```python
from build123d import *

# Parameters (mm, degrees)
SKETCH2_R            = 39.5
BOSS_EXTRUDE1_DEPTH  = 1
SKETCH4_R            = 41.25
BOSS_EXTRUDE2_DEPTH  = 0.7
SKETCH5_R            = 42
BOSS_EXTRUDE3_DEPTH  = 7
SKETCH6_R            = 35
BOSS_EXTRUDE4_DEPTH  = 3
SKETCH7_R            = 2.959266208
BOSS_EXTRUDE5_DEPTH  = 2.7
SKETCH8_R            = 2.259266208
CUT_EXTRUDE1_DEPTH   = 0.5
CIRPATTERN1_COUNT    = 12
SKETCH9_W            = 24
SKETCH9_H            = 40
BOSS_EXTRUDE6_DEPTH  = 42
BOSS_EXTRUDE7_DEPTH  = 24
SKETCH13_R           = 10
BOSS_EXTRUDE10_DEPTH = 10
SKETCH14_R           = 10
BOSS_EXTRUDE11_DEPTH = 10


with BuildPart() as part:
    # Sketch1 → Revolve1 (revolve)
    with BuildSketch(Plane.XY, mode=Mode.PRIVATE) as revolve1_sk:
        with BuildLine():
            Line((0, 0), (-35, 0))
            ThreePointArc((-35, 0), (-39.657515479, -9.46062113), (-40, -20))
            Line((-40, -20), (0, -20))
            Line((0, -20), (0, 0))
        make_face()
    revolve(revolve1_sk.sketch.rotate(Axis((0, 0, 0), (0, -1, 0)), 270), axis=Axis((0, 0, 0), (0, -1, 0)))

    # Sketch2 → Boss-Extrude1 (add)
    with BuildSketch(Plane.XZ.offset(20)):
        with Locations(Location((0, 0, 0), (0, 0, 270))):
            Circle(SKETCH2_R)
    extrude(amount=BOSS_EXTRUDE1_DEPTH)

    # Sketch3 → Revolve2 (revolve)
    with BuildSketch(Plane.XY, mode=Mode.PRIVATE) as revolve2_sk:
        with BuildLine():
            Line((0, -21), (-40, -21))
            ThreePointArc((-40, -21), (-42.384109041, -30.861589096), (-42, -41))
            Line((-42, -41), (0, -41))
            Line((0, -41), (0, -21))
        make_face()
    revolve(revolve2_sk.sketch.rotate(Axis((0, -21, 0), (0, -1, 0)), 270), axis=Axis((0, -21, 0), (0, -1, 0)))

    # Sketch4 → Boss-Extrude2 (add)
    with BuildSketch(Plane.XZ.offset(41)):
        Circle(SKETCH4_R)
    extrude(amount=BOSS_EXTRUDE2_DEPTH)

    # Sketch5 → Boss-Extrude3 (add)
    with BuildSketch(Plane.XZ.offset(41.7)):
        Circle(SKETCH5_R)
    extrude(amount=BOSS_EXTRUDE3_DEPTH)

    # Sketch6 → Boss-Extrude4 (add)
    with BuildSketch(Plane.XZ.offset(48.7)):
        Circle(SKETCH6_R)
    extrude(amount=BOSS_EXTRUDE4_DEPTH)

    # Sketch7 → Boss-Extrude5 (add)
    with BuildSketch(Plane.XZ.offset(48.7)):
        with Locations(Location((38.5, 0, 0), (0, 0, 180))):
            Circle(SKETCH7_R)
    boss_extrude5 = extrude(amount=BOSS_EXTRUDE5_DEPTH)

    # Sketch8 → Cut-Extrude1 (cut)
    with BuildSketch(Plane.XZ.offset(51.4)):
        with Locations((38.5, 0)):
            Circle(SKETCH8_R)
    cut_extrude1 = extrude(amount=-CUT_EXTRUDE1_DEPTH, mode=Mode.SUBTRACT)

    # CirPattern1: Boss-Extrude5, Cut-Extrude1 ×12 about axis
    cirpattern1_axis = Axis((0, 0, 0), (0, 1, 0))
    add([boss_extrude5.rotate(cirpattern1_axis, i * 360 / CIRPATTERN1_COUNT) for i in range(1, CIRPATTERN1_COUNT)])
    add([cut_extrude1.rotate(cirpattern1_axis, i * 360 / CIRPATTERN1_COUNT) for i in range(1, CIRPATTERN1_COUNT)], mode=Mode.SUBTRACT)

    # Sketch9 → Boss-Extrude6 (add)
    with BuildSketch(Plane(origin=(0, 0, 0), x_dir=(1, 0, 0), z_dir=(0, 1, 0))):
        Rectangle(SKETCH9_W, SKETCH9_H)
    extrude(amount=BOSS_EXTRUDE6_DEPTH)

    # Sketch10 → Boss-Extrude7 (add)
    with BuildSketch(Plane(origin=(12, 0, 0), x_dir=(0, 0, -1), z_dir=(1, 0, 0))):
        with BuildLine():
            Line((-20, 42), (20, 42))
            ThreePointArc((20, 42), (0, 62), (-20, 42))
        make_face()
    extrude(amount=-BOSS_EXTRUDE7_DEPTH)

    # Sketch13 → Boss-Extrude10 (add)
    with BuildSketch(Plane.ZY.offset(12)):
        with Locations(Location((0, 42, 0), (0, 0, 180))):
            Circle(SKETCH13_R)
    extrude(amount=BOSS_EXTRUDE10_DEPTH)

    # Sketch14 → Boss-Extrude11 (add)
    with BuildSketch(Plane.XZ.offset(51.7)):
        Circle(SKETCH14_R)
    extrude(amount=BOSS_EXTRUDE11_DEPTH)


solid = part.part
```
CAD build for the part. Positions are in the model's coordinates, mm. A direction names the side the tool comes from. Round coordinates to 2 decimals unless told otherwise and drop trailing zeros. Order: outer loops, then holes, each group sorted by start corner. A loop starts at its lowest first (then second) coordinate and runs counter-clockwise, first axis right, second up. Notation, with made-up numbers: (-25, -14.5) -> (16, -14.5) arc R18 ccw to (16, -8.5) -> close; hole circle Ø2 at (19, -19.5). An arc over 180 degrees is marked (long way). Write item = value, one per line.
(1) Cut at A-A (y = 48). Write the cut outline in (x, z), plus the area to 3 significant figures.
Answers follow:
outline = (-22, -8) -> (-12, -8) -> (-12, -19.08) -> (12, -19.08) -> (12, 19.08) -> (-12, 19.08) -> (-12, 8) -> (-22, 8) -> close
area = 1,080 mm²
(2) Pull direction X, two halves, no side cores. Call faces 1 (the cylindrical face through (-33.441, -51.154, -21.507)), 2 (the flat face through (38.73, -51.4, 2.4)), 3 (the flat face through (-22, 42, 0)), 4 (the cylindrical face through (-40.655, -51.154, -0.679)): +X half, -X half, draft (parallel to the pull), parting line (faces both ways), or undercut.
Answers follow:
face_1 = undercut
face_2 = draft
face_3 = -X half
face_4 = undercut
(3) 3-axis set-ups, long thin cutter, end or side, ignore diameter. For faces 5 (the flat face through (-19, -51.4, -36)), 6 (the flat face through (-21, -51.4, 35)), 7 (the flat face through (31, -41, 28)), 8 (the cylindrical face through (-30.453, -50.031, 18.608)): which of +Z, -Z, +X, -X, +Y, -Y reach the whole face in a straight line?
Answers follow:
face_5 = -Z, -X, -Y
face_6 = +Z, -X, -Y
face_7 = none
face_8 = -Y
(4) Drill centre lines: L1, parallel to X at y = -51, z = -19; L2, parallel to Y at x = -14, z = -25; L3, parallel to Z at x = 38.5, y = -51.15. Where is each one in solid material? Low to high.
Answers follow:
L1 = -36.29 to -35.59, -31.1 to -30.39, -29.39 to 29.39, 30.39 to 31.1, 35.59 to 36.29
L2 = -51.7 to 0
L3 = -2.96 to -2.26, 2.26 to 2.96
(5) Flat gauge pins, fed straight in: P1, Ø4, axis at x = 16, y = -8, coming from the +Z side; P2, Ø5, axis at x = 32.5, z = 19, coming from the -Y side; P3, Ø2.5, axis at x = 0, z = -38.5, coming from the -Y side. Where does each tip first touch, or does it go through?
Answers follow:
P1 = 36.88
P2 = -51.4
P3 = -50.9
(6) Cut at B-B (y = -44.5). Write the cut outline in (x, z), plus the area to 3 significant figures.
Answers follow:
outline = circle Ø84 at (0, 0)
area = 5,540 mm²
